Work out the finished part from the listing and answer in its coordinate system (mm). A direction names the side the tool comes from. Coordinates: 2 decimals unless noted, no trailing zeros. Loops run counter-clockwise (first coordinate to the right, second up) from the corner with the lowest first, then second, coordinate; pieces in that order, holes last.
```python
from build123d import *

# Parameters (mm, degrees)
SKETCH1_R           = 50
BOSS_EXTRUDE1_DEPTH = 10
SKETCH3_R           = 8
CUT_EXTRUDE1_DEPTH  = 20
SKETCH4_R           = 1.5
CUT_EXTRUDE2_DEPTH  = 30
SKETCH5_R           = 1
CUT_EXTRUDE3_DEPTH  = 10


with BuildPart() as part:
    # Sketch1 → Boss-Extrude1 (new body)
    with BuildSketch(Plane.XY):
        Circle(SKETCH1_R)
        with BuildLine():
            Line((17.67766953, -17.67766953), (-17.67766953, -17.67766953))
            ThreePointArc((-17.67766953, -17.67766953), (0, 25), (17.67766953, -17.67766953))
        make_face(mode=Mode.SUBTRACT)
    extrude(amount=BOSS_EXTRUDE1_DEPTH)

    # Sketch3 → Cut-Extrude1 (cut)
    with BuildSketch(Plane(origin=(0, 0, 0), x_dir=(-1, 0, 0), z_dir=(0, 0, -1))):
        with Locations((-14.146357726, 34.109474384)):
            Circle(SKETCH3_R)
        with Locations((14.116055163, 34.122026117)):
            Circle(SKETCH3_R)
        with Locations((34.109474384, 14.146357726)):
            Circle(SKETCH3_R)
        with Locations((34.122026117, -14.116055163)):
            Circle(SKETCH3_R)
        with Locations((14.146357726, -34.109474384)):
            Circle(SKETCH3_R)
        with Locations((-14.116055163, -34.122026117)):
            Circle(SKETCH3_R)
        with Locations((-34.109474384, -14.146357726)):
            Circle(SKETCH3_R)
        with Locations((-34.122026117, 14.116055163)):
            Circle(SKETCH3_R)
    extrude(amount=-CUT_EXTRUDE1_DEPTH, mode=Mode.SUBTRACT)

    # Sketch4 → Cut-Extrude2 (cut)
    with BuildSketch(Plane(origin=(0, 0, 0), x_dir=(-1, 0, 0), z_dir=(0, 0, -1))):
        with Locations((0, 46.99)):
            Circle(SKETCH4_R)
        with Locations((46.99, 0)):
            Circle(SKETCH4_R)
        with Locations((0, -46.99)):
            Circle(SKETCH4_R)
        with Locations((-46.99, 0)):
            Circle(SKETCH4_R)
    extrude(amount=-CUT_EXTRUDE2_DEPTH, mode=Mode.SUBTRACT)

    # Sketch5 → Cut-Extrude3 (cut)
    with BuildSketch(Plane(origin=(0, -17.67766953, 0), x_dir=(1, 0, 0), z_dir=(0, 1, 0))):
        with Locations(Location((10, -7.5, 0), (0, 0, 180))):
            Circle(SKETCH5_R)
        with Locations(Location((-10, -7.5, 0), (0, 0, 180))):
            Circle(SKETCH5_R)
    extrude(amount=-CUT_EXTRUDE3_DEPTH, mode=Mode.SUBTRACT)


solid = part.part
```
1. Each of these flat-tipped pins is pushed along its axis until it touches: P1, Ø5, axis at y = 11.5, z = 4.5, coming from the +X side; P2, Ø1.6, axis at x = 10, z = 7.5, coming from the -Y side; P3, Ø3, axis at x = 8, z = 6.5, coming from the +Y side. Where does it stop, or does it pass through?
2. Straight lines are drawn through the part: probe 1 along Y at (x, z) = (0, 6); probe 2 along Y at (x, z) = (-34.5, 8); probe 3 along Y at (x, z) = (-12.5, 5.5). For each, find the intervals that lie inside material, in ascending order.
3. A cutting plane is placed at A-A, the plane x = 0. Give the vertices of the cut face in (y, z).
4. A cutting plane is placed at D-D, the plane y = 29. Give the vertices of the cut face in (x, z).
5. Determine the mould class of faces 3 (the cylindrical face through (15.85, -41.93, 4.93)), 4 (the cylindrical face through (47.69, 15.02, 4.93)), 5 (the flat face through (-1, -22, 0)), 6 (the cylindrical face through (-18.417, 40.868, 4.93)) for opening direction X: released by +X, released by -X, zero draft, split by the parting line, or undercut.
6. A cutting plane is placed at C-C, the plane x = 32. Give the vertices of the cut face in (y, z), then the cut area to 3 significant figures.
7. For faces 1 (the flat face through (-1, -22, 10)), 2 (the flat face through (0, -17.678, 5)), determine the directions among +Z, -Z, +X, -X, +Y, -Y from which every point of the face is accessible in a straight line to the end or side of a thin tool.
8. A cutting plane is placed at B-B, the plane y = 0. Give the vertices of the cut face in (x, z).
Answers below:
1. P1: stops at x = 49.18
1. P2: stops at y = -49.15
1. P3: stops at y = 49.58
2. probe 1: y = -50 to -48.49, -45.49 to -17.68, 25 to 45.49, 48.49 to 50
2. probe 2: y = -36.19 to -22.11, -6.12 to 6.16, 22.14 to 36.19
2. probe 3: y = -48.41 to -41.94, -26.28 to -17.68, 21.65 to 26.29, 41.96 to 48.41
3. outline: (-50, 0) - (-48.49, 0) - (-48.49, 10) - (-50, 10) - close; (-45.49, 0) - (-17.68, 0) - (-17.68, 10) - (-45.49, 10) - close; (25, 0) - (45.49, 0) - (45.49, 10) - (25, 10) - close; (48.49, 0) - (50, 0) - (50, 10) - (48.49, 10) - close
4. outline: (-40.73, 0) - (-20.26, 0) - (-20.26, 10) - (-40.73, 10) - close; (-7.97, 0) - (7.99, 0) - (7.99, 10) - (-7.97, 10) - close; (20.3, 0) - (40.73, 0) - (40.73, 10) - (20.3, 10) - close
5. face 3: undercut
5. face 4: split by the parting line
5. face 5: zero draft
5. face 6: undercut
6. outline: (-38.42, 0) - (-21.86, 0) - (-21.86, 10) - (-38.42, 10) - close; (-6.43, 0) - (6.4, 0) - (6.4, 10) - (-6.43, 10) - close; (21.83, 0) - (38.42, 0) - (38.42, 10) - (21.83, 10) - close
6. area: 460 mm2
7. face 1: +Z, +X, -X, +Y, -Y
7. face 2: +Z, -Z
8. outline: (-50, 0) - (-48.49, 0) - (-48.49, 10) - (-50, 10) - close; (-45.49, 0) - (-25, 0) - (-25, 10) - (-45.49, 10) - close; (25, 0) - (45.49, 0) - (45.49, 10) - (25, 10) - close; (48.49, 0) - (50, 0) - (50, 10) - (48.49, 10) - close
